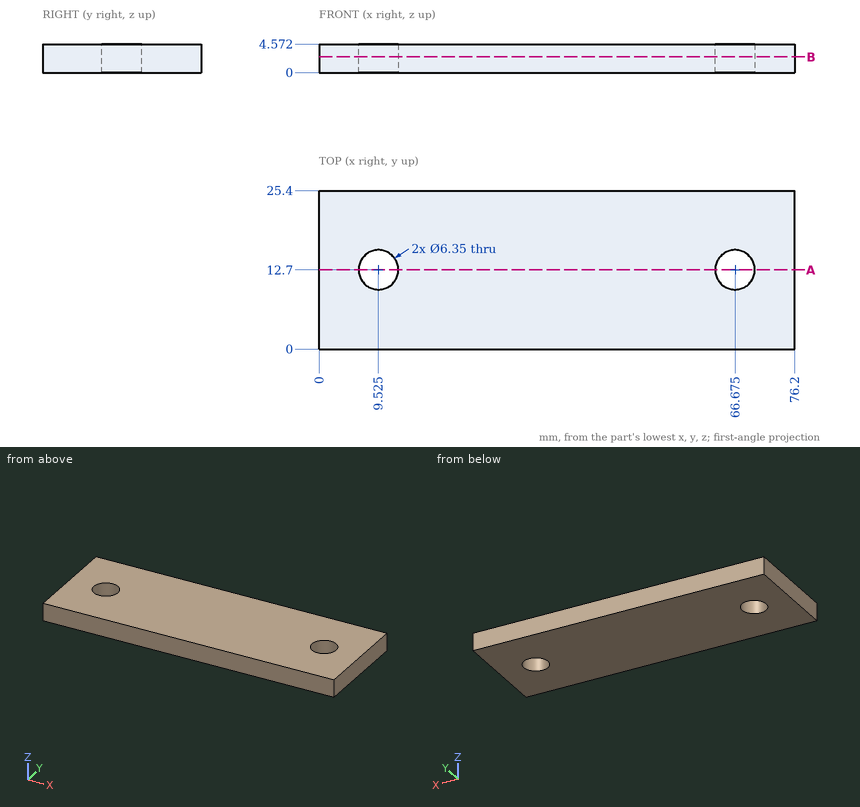
The figure shows three views and two pictorial views of one solid part (mm, origin at its lowest corner). Answer the questions. Coordinates: 2 decimals unless noted, no trailing zeros. Write each loop counter-clockwise with the first axis right and the second up, starting at its lowest first coordinate (ties: lowest second). Pieces come first, ordered by that corner, then holes.
1. The part is cut by section B-B, the plane z = 2.5. Write down the section's boundary in (x, y) (3 decimals), and give its area (3 significant figures).
Results list:
outline: (0, 0) - (76.2, 0) - (76.2, 25.4) - (0, 25.4) - close; hole circle Ø6.35 at (9.525, 12.7); hole circle Ø6.35 at (66.675, 12.7)
area: 1,870 mm2
2. Consider line 1 along X through (y, z) = (11.25, 3.95); line 2 along X through (y, z) = (12, 2.3); line 3 along Y through (x, z) = (65, 2.6). Determine where each line is inside the solid, lowest interval first.
Results list:
line 1: x = 0 to 6.7, 12.35 to 63.85, 69.5 to 76.2
line 2: x = 0 to 6.43, 12.62 to 63.58, 69.77 to 76.2
line 3: y = 0 to 10, 15.4 to 25.4
3. The part is cut by section A-A, the plane y = 12.7. Write down the section's boundary in (x, z), and give its area (3 significant figures).
Results list:
outline: (0, 0) - (6.35, 0) - (6.35, 4.57) - (0, 4.57) - close; (12.7, 0) - (63.5, 0) - (63.5, 4.57) - (12.7, 4.57) - close; (69.85, 0) - (76.2, 0) - (76.2, 4.57) - (69.85, 4.57) - close
area: 290 mm2
